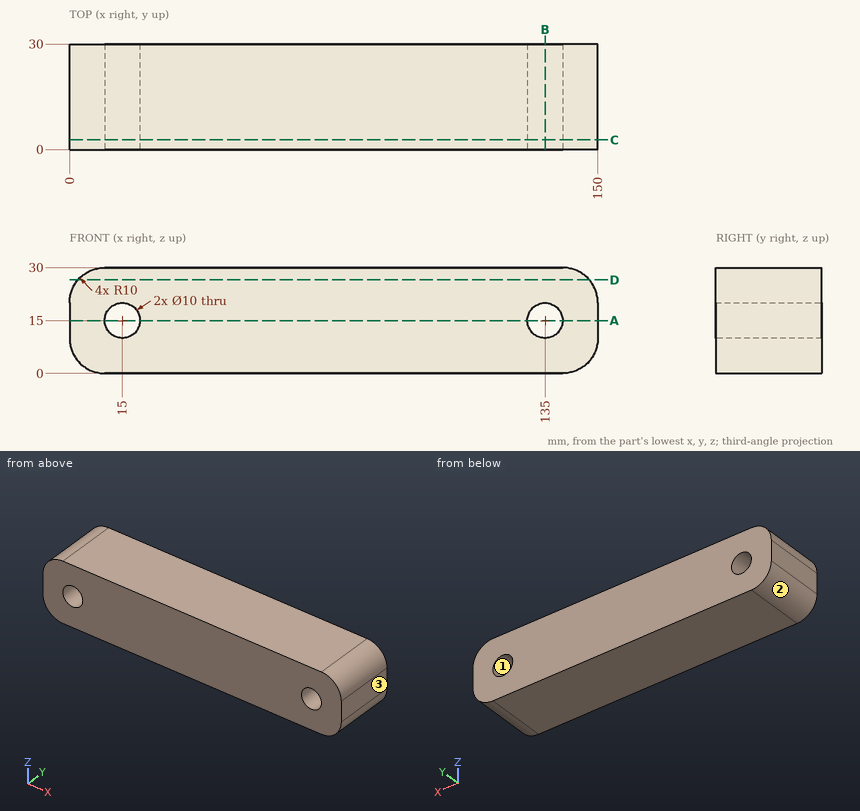
Part print with two shaded views. Sizes in mm from the minimum x, y, z corner. Round coordinates to 2 decimals unless told otherwise and drop trailing zeros. Order: outer loops, then holes, each group sorted by start corner. A loop starts at its lowest first (then second) coordinate and runs counter-clockwise, first axis right, second up. Notation, with made-up numbers: M -4,60 L 42,60 A17 cw 42,74 Z; hole C 22.5,-34 d6. An arc over 180 degrees is marked long. Use CSV: the item, a comma, the result in double quotes. Start each with the question number.
(1) Flat gauge pin, fed straight in: P1, Ø1.5, axis at y = 11, z = 4, coming from the -X side. Where does the tip first touch, or does it go through?
(2) Cut at A-A on z = 15. List the corners of the cut face in (x, y).
(3) Mould opens along Z. For the marked faces 1, 2 and 3 say: +Z half, -Z half, draft (parallel to the pull), parting line (faces both ways), or undercut.
(4) Drill centre lines: probe 1 along X at (y, z) = (13.5, 15); probe 2 along X at (y, z) = (12, 10.5); probe 3 along Z at (x, y) = (135, 17). Where is each one in solid material? Low to high.
(5) Cut at D-D on z = 26.5. List the corners of the cut face in (x, y).
(6) Cut at C-C on y = 2.75. List the corners of the cut face in (x, z).
(7) Cut at B-B on x = 135. List the corners of the cut face in (y, z), then the cut area to 3 significant figures.
Findings:
1,P1,"stops at x = 1.49"
2,outline,"M 0,0 L 10,0 L 10,30 L 0,30 Z; M 20,0 L 130,0 L 130,30 L 20,30 Z; M 140,0 L 150,0 L 150,30 L 140,30 Z"
3,face 1,"undercut"
3,face 2,"-Z half"
3,face 3,"draft"
4,probe 1,"x = 0 to 10, 20 to 130, 140 to 150"
4,probe 2,"x = 0 to 12.82, 17.18 to 132.82, 137.18 to 150"
4,probe 3,"z = 0 to 10, 20 to 30"
5,outline,"M 2.4,0 L 147.6,0 L 147.6,30 L 2.4,30 Z"
6,outline,"M 0,10 A10 ccw 10,0 L 140,0 A10 ccw 150,10 L 150,20 A10 ccw 140,30 L 10,30 A10 ccw 0,20 Z; hole C 15,15 d10; hole C 135,15 d10"
7,outline,"M 0,0 L 30,0 L 30,10 L 0,10 Z; M 0,20 L 30,20 L 30,30 L 0,30 Z"
7,area,"600 mm^2"
